from build123d import *

# Parameters (mm, degrees)
EXTRUDE_1_DEPTH     = 80
SKETCH_10_W         = 4
SKETCH_10_H         = 8
EXTRUDE_8_DEPTH     = 80
EXTRUDE_9_DEPTH     = 4
SKETCH_12_W         = 70
SKETCH_12_H         = 40.815900945
CUT_EXTRUDE_1_DEPTH = 10
SKETCH_13_W         = 5
SKETCH_13_H         = 4
CUT_EXTRUDE_2_DEPTH = 10


with BuildPart() as part:
    # 草图1 → 凸台-拉伸1 (new body)
    with BuildSketch(Plane(origin=(0, 0, 0), x_dir=(0, 0, -1), z_dir=(1, 0, 0))):
        with BuildLine():
            Line((-18, 2), (18, 2))
            Line((18, 2), (20, 2))
            Line((20, 2), (20, 0))
            ThreePointArc((20, 0), (19.414213562, -1.414213562), (18, -2))
            Line((18, -2), (-18, -2))
            ThreePointArc((-18, -2), (-20, 0), (-18, 2))
        make_face()
    extrude(amount=EXTRUDE_1_DEPTH)

    # 草图10 → 凸台-拉伸8 (add)
    with BuildSketch(Plane(origin=(80, 0, 0), x_dir=(0, 0, -1), z_dir=(1, 0, 0))):
        with Locations((18, 6)):
            Rectangle(SKETCH_10_W, SKETCH_10_H)
    extrude(amount=-EXTRUDE_8_DEPTH)

    # 草图11 → 凸台-拉伸9 (add)
    with BuildSketch(Plane(origin=(0, 0, -20), x_dir=(-1, 0, 0), z_dir=(0, 0, -1))):
        with BuildLine():
            Line((-6, 10), (-14, 10))
            Line((-14, 10), (-14, 18))
            ThreePointArc((-14, 18), (-10, 22), (-6, 18))
            Line((-6, 18), (-6, 10))
        make_face()
        with BuildLine():
            Line((-72, 6), (-80, 6))
            Line((-80, 6), (-80, 10))
            ThreePointArc((-80, 10), (-76, 14), (-72, 10))
            Line((-72, 10), (-72, 6))
        make_face()
    extrude(amount=-EXTRUDE_9_DEPTH)

    # 草图12 → 切除-拉伸1 (cut)
    with BuildSketch(Plane(origin=(0, 2, 0), x_dir=(1, 0, 0), z_dir=(0, 1, 0))):
        with Locations((40, -4.407950473)):
            Rectangle(SKETCH_12_W, SKETCH_12_H)
    extrude(amount=-CUT_EXTRUDE_1_DEPTH, mode=Mode.SUBTRACT)

    # 草图13 → 切除-拉伸2 (cut)
    with BuildSketch(Plane.XY.offset(-16)):
        with Locations((7.5, 0)):
            Rectangle(SKETCH_13_W, SKETCH_13_H)
        with Locations((72.5, 0)):
            Rectangle(SKETCH_13_W, SKETCH_13_H)
    extrude(amount=-CUT_EXTRUDE_2_DEPTH, mode=Mode.SUBTRACT)


solid = part.part
Can you work these out from the model? Positions are in its coordinate system, mm. A direction names the side the tool comes from. Coordinates: 2 decimals unless noted, no trailing zeros. Loops run counter-clockwise (first coordinate to the right, second up) from the corner with the lowest first, then second, coordinate; pieces in that order, holes last. Notation, with made-up numbers: (-21.75, -34.75) - (18.25, -34.75) arc R31 cw to (18.25, -3.75) - close; hole circle Ø6 at (18, -21.5). An arc over 180 degrees is marked (long way). Answer as a JSON object with one key per item and string values. Group by question number.
Item 1: If we section it at D-D (z = -17): List the corners of the cut face in (x, y) for me.
Item 2: For pin 1 (1.2 mm diameter, centred on x = 41.5, z = -19, fed in from +Y); pin 2 (4.5 mm diameter, centred on y = 13.5, z = -18, fed in from -X); pin 3 (1.5 mm diameter, centred on x = 77.5, z = -5.5, fed in from +Y), each with a flat end and sliding along its axis, tell me the tip position at first contact or that it passes through.
Item 3: If we mould it in two halves opening along X, with no side actions, what happens to faces 1 (the face through (7, 2, -18)), 2 (the face through (0, 1, -4)), 3 (the face through (2, -2, 0))? For each: released by +X, released by -X, zero draft, split by the parting line, or undercut.
Item 4: If we section it at B-B (y = 11.75): List the corners of the cut face in (x, z) for me, plus the area to 3 significant figures.
Item 5: On a 3-axis mill with a long thin cutter (end or side, diameter ignored), from which of +Z, -Z, +X, -X, +Y, -Y can I reach the whole of each face in a straight line? I mean faces 4 (the face through (2, 2, 1)), 5 (the face through (70, 0, -18)), 6 (the face through (3, 10, -18)), 7 (the face through (14, 14, -18)), 8 (the face through (41, 6, -20)). Say none if no direction works.
Item 6: If I drill on L1, parallel to X at y = 0.5, z = -17.5; L2, parallel to X at y = -0.25, z = 8.5; L3, parallel to Z at x = 70, y = 5.75, over which ranges is the centre line in solid material (lowest first)? Write a range as from..to.
Item 7: If we section it at A-A (z = -1): List the corners of the cut face in (x, y) for me, plus the area to 3 significant figures.
Item 8: If we section it at C-C (x = 76): List the corners of the cut face in (y, z) for me, plus the area to 3 significant figures.
Returned:
{
 "1": {"outline": "(0, -2) - (5, -2) - (5, 2) - (10, 2) - (10, -2) - (70, -2) - (70, 2) - (75, 2) - (75, -2) - (80, -2) - (80, 10) arc R4 ccw to (72, 10) - (14, 10) - (14, 18) arc R4 ccw to (6, 18) - (6, 10) - (0, 10) - close"},
 "2": {"pin 1": "stops at y = 10", "pin 2": "stops at x = 6", "pin 3": "stops at y = 2"},
 "3": {"face 1": "undercut", "face 2": "released by -X", "face 3": "zero draft"},
 "4": {"outline": "(6, -20) - (14, -20) - (14, -16) - (6, -16) - close; (72.4, -20) - (79.6, -20) - (79.6, -16) - (72.4, -16) - close", "area": "60.8 mm²"},
 "5": {"face 4": "+Z, +X, -X, +Y", "face 5": "+Z, -Z, -Y", "face 6": "+Z, -Z, -X, +Y", "face 7": "+Z, -Z, +Y", "face 8": "-Z, +X, -X, +Y, -Y"},
 "6": {"L1": "x = 0..5, 10..70, 75..80", "L2": "x = 0..5, 75..80", "L3": "z = -20..-16"},
 "7": {"outline": "(0, -2) - (5, -2) - (5, 2) - (0, 2) - close; (75, -2) - (80, -2) - (80, 2) - (75, 2) - close", "area": "40.0 mm²"},
 "8": {"outline": "(-2, -18) arc R2 ccw to (0, -20) - (14, -20) - (14, -16) - (2, -16) - (2, 18) arc R2 ccw to (-2, 18) - close", "area": "205 mm²"}
}
